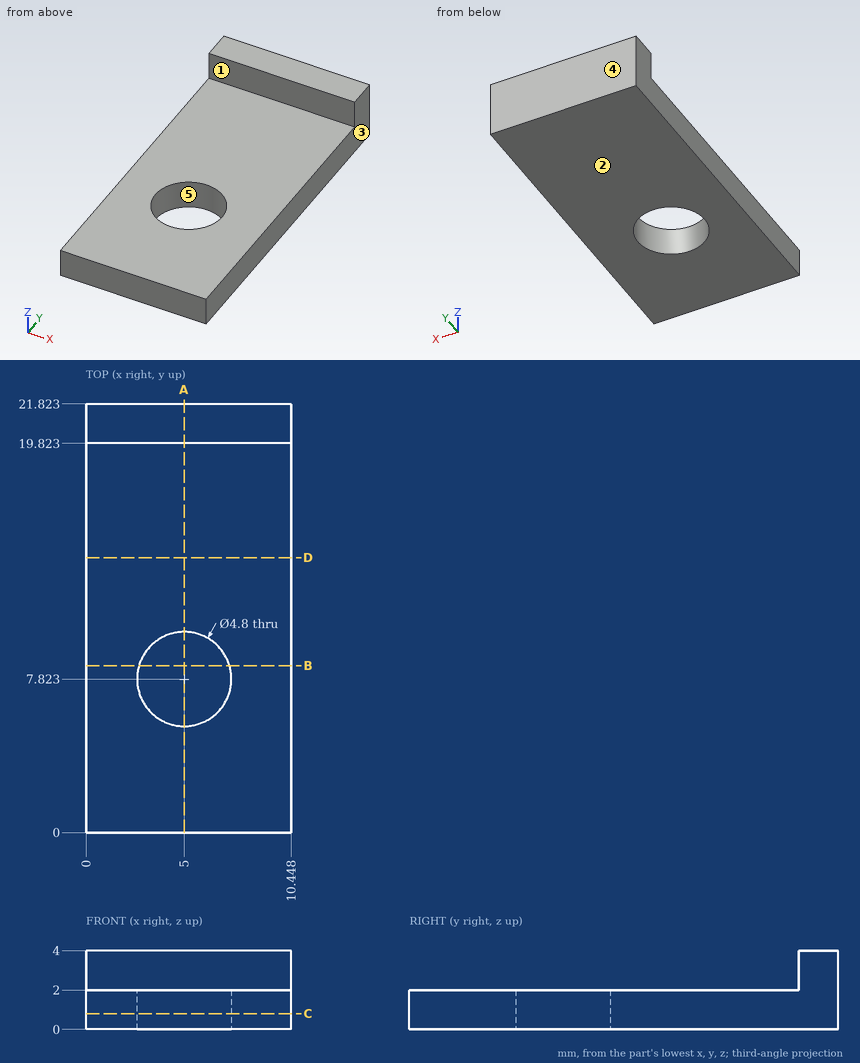
Print and shaded views of the part. All mm, measured from the part's lowest x, y and z. A direction names the side the tool comes from. Coordinates: 2 decimals unless noted, no trailing zeros. Order: outer loops, then holes, each group sorted by start corner. A loop starts at its lowest first (then second) coordinate and runs counter-clockwise, first axis right, second up. Notation, with made-up numbers: (30, 81) -> (76, 81) arc R29 ccw to (76, 103) -> close; hole circle Ø8 at (-30.75, -13). An arc over 180 degrees is marked (long way). Answer as a JSON object with one key per item and string values. Group by question number.
1) Drill centre lines: L1, parallel to Y at x = 5, z = 1.5; L2, parallel to Z at x = 2.5, y = 3.75; L3, parallel to Y at x = 1.75, z = 3.6. Where is each one in solid material? Low to high.
2) Cut at B-B, the plane y = 8.5. Write the cut outline in (x, z), then the cut area to 3 significant figures.
3) Cut at D-D, the plane y = 14. Write the cut outline in (x, z), then the cut area to 3 significant figures.
4) Pull direction X, two halves, no side cores. Call the marked faces 3, 4 and 5: +X half, -X half, draft (parallel to the pull), parting line (faces both ways), or undercut.
5) Cut at A-A, the plane x = 5. Write the cut outline in (y, z).
6) Flat gauge pins, fed straight in: pin 1 (4 mm diameter, centred on x = 5, y = 7.82, fed in from -Z); pin 2 (0.6 mm diameter, centred on x = 4, z = 2.5, fed in from -Y). Where does each tip first touch, or does it go through?
7) Cut at C-C, the plane z = 0.8. Write the cut outline in (x, y), then the cut area to 3 significant figures.
8) Which spindle directions (+Z, -Z, +X, -X, +Y, -Y) get a long thin tool onto all of the face, cutting with end or side? Do the marked faces 1 and 2. Say none if no direction does.
Check values:
{
 "1": {"L1": "y = 0 to 5.42, 10.22 to 21.82", "L2": "z = 0 to 2", "L3": "y = 19.82 to 21.82"},
 "2": {"outline": "(0, 0) -> (2.7, 0) -> (2.7, 2) -> (0, 2) -> close; (7.3, 0) -> (10.45, 0) -> (10.45, 2) -> (7.3, 2) -> close", "area": "11.7 mm²"},
 "3": {"outline": "(0, 0) -> (10.45, 0) -> (10.45, 2) -> (0, 2) -> close", "area": "20.9 mm²"},
 "4": {"face 3": "+X half", "face 4": "draft", "face 5": "undercut"},
 "5": {"outline": "(0, 0) -> (5.42, 0) -> (5.42, 2) -> (0, 2) -> close; (10.22, 0) -> (21.82, 0) -> (21.82, 4) -> (19.82, 4) -> (19.82, 2) -> (10.22, 2) -> close"},
 "6": {"pin 1": "passes through", "pin 2": "stops at y = 19.82"},
 "7": {"outline": "(0, 0) -> (10.45, 0) -> (10.45, 21.82) -> (0, 21.82) -> close; hole circle Ø4.8 at (5, 7.82)", "area": "210 mm²"},
 "8": {"face 1": "+Z, +X, -X, -Y", "face 2": "-Z, +X, -X, +Y, -Y"}
}
